from build123d import *

# Parameters (mm, degrees)
F0_W     = 100
F0_H     = 40
F1_DEPTH = 20
F2_SIZE  = 12.7
F3_W     = 14.7754922509
F3_H     = 3
F4_DEPTH = 25
F5_W     = 70
F5_H     = 10
F6_DEPTH = 5


with BuildPart() as f1:
    # F0 (on Front) → F1 (new body)
    with BuildSketch(Plane.XZ):
        with Locations((-20.0241699815, -7.6543013752)):
            Rectangle(F0_W, F0_H)
    extrude(amount=F1_DEPTH)

    # F2
    f2_edges = [f1.edges().sort_by_distance(p)[0] for p in [
        (-70.02417, -20, -7.654301),
        (29.97583, -20, -7.654301),
        (-20.02417, -20, -27.654301),
        (-20.02417, -20, 12.345699),
    ]]
    chamfer(f2_edges, length=F2_SIZE)

    # F3 (on face) → F4 (cut)
    with BuildSketch(Plane(origin=(0, -9.8228493124, 9.8228493124), x_dir=(1, 0, 0), z_dir=(0, -0.7071067812, 0.7071067812))):
        with Locations((-49.1398386657, -1.5)):
            Rectangle(F3_W, F3_H)
    extrude(amount=-F4_DEPTH, mode=Mode.SUBTRACT)

    # F5 (on face) → F6 (cut)
    with BuildSketch(Plane.XZ.offset(20)):
        with Locations((-20.430685021, -7.0188848879)):
            Rectangle(F5_W, F5_H)
    extrude(amount=-F6_DEPTH, mode=Mode.SUBTRACT)


solid = f1.part
The model under review builds one solid part; all positions refer to its coordinate system, in mm. A direction names the side the tool comes from. Coordinates: 2 decimals unless noted, no trailing zeros. Loops run counter-clockwise (first coordinate to the right, second up) from the corner with the lowest first, then second, coordinate; pieces in that order, holes last.
(1) Tool access review of faces 4 (the flat face through (-21, -18, -2.019)), 5 (the flat face through (-49.243, -6.056, 1.813)), 6 (the flat face through (-21, -4, -27.654)): name each direction out of +Z, -Z, +X, -X, +Y, -Y from which nothing blocks a thin tool from reaching the whole face with its end or side.
Determined:
face 4: -Y
face 5: none
face 6: -Z, +X, -X, +Y, -Y
(2) Consider section D-D, the plane y = -11. Give the boundary of the cut face in (x, z), plus the area to 3 significant figures.
Determined:
outline: (-66.32, -23.95) - (26.28, -23.95) - (26.28, 8.65) - (-41.75, 8.65) - (-41.75, 6.76) - (-56.53, 6.76) - (-56.53, 8.65) - (-66.32, 8.65) - close
area: 2,990 mm2
(3) Consider section A-A, the plane x = -43. Give the boundary of the cut face in (y, z).
Determined:
outline: (-20, -14.95) - (-7.3, -27.65) - (0, -27.65) - (0, -4.24) - (-11.94, 7.7) - (-20, -0.35) - (-20, -2.02) - (-15, -2.02) - (-15, -12.02) - (-20, -12.02) - close; (-9.82, 9.82) - (0, 0) - (0, 12.35) - (-7.3, 12.35) - close
(4) Draft analysis for pull direction X (two halves, no side actions). For faces 1 (the flat face through (-64.996, -12.328, -7.934)), 2 (the flat face through (-20.2, -20, -12.5)), 3 (the flat face through (-49, -5, 5)), state which applies: +X half, -X half, draft (parallel to the pull), parting line (faces both ways), or undercut.
Determined:
face 1: -X half
face 2: draft
face 3: undercut
(5) Insertion check: P1, Ø8, axis at x = -35, y = -14, coming from the -Z side; P2, Ø1.5, axis at y = -17.5, z = -6, coming from the -X side; P3, Ø1.5, axis at x = -35, y = -17.5, coming from the -Z side. Each pin has a flat end and moves straight along its axis. Give the tip position at first contact, or say it passes through.
Determined:
P1: stops at z = -24.95
P2: stops at x = -60.57
P3: stops at z = -18.2
(6) Wall thickness on L1, parallel to Z at x = 1.5, y = -18.5; L2, parallel to Y at x = -39.5, z = -5; L3, parallel to Z at x = -7, y = -11.5: over which ranges is each line inside the solid? List them lowest first.
Determined:
L1: z = -16.45 to -12.02, -2.02 to 1.15
L2: y = -15 to 0
L3: z = -23.45 to 8.15
(7) Consider section B-B, the plane z = 1. Give the boundary of the cut face in (x, y).
Determined:
outline: (-70.02, -7.3) - (-58.68, -18.65) - (18.63, -18.65) - (29.98, -7.3) - (29.98, 0) - (-70.02, 0) - close; hole (-56.53, -5.24) - (-41.75, -5.24) - (-41.75, -1) - (-56.53, -1) - close
(8) Consider section C-C, the plane y = -17. Give the boundary of the cut face in (x, z).
Determined:
outline: (-60.32, -17.95) - (20.28, -17.95) - (20.28, 2.65) - (-60.32, 2.65) - close; hole (-55.43, -12.02) - (14.57, -12.02) - (14.57, -2.02) - (-55.43, -2.02) - close
